Part print with two shaded views. Sizes in mm from the minimum x, y, z corner. Round coordinates to 2 decimals unless told otherwise and drop trailing zeros. Loops run counter-clockwise (first coordinate to the right, second up) from the corner with the lowest first, then second, coordinate; pieces in that order, holes last. Notation, with made-up numbers: M 71,65.25 L 91,65.25 A15 ccw 91,84.25 Z; hole C 63.5,-37.75 d7. An arc over 180 degrees is marked long. Answer as CSV lines item,"result". Start each with the question number.
Item 1: Band-saw the part on B-B (y = 2.2). Count the separate pieces of the cut face and the enclosed holes in it, and give its area (3 significant figures).
Item 2: Wall check: line 1 (X direction, y = 2.4, z = 103.6); line 2 (X direction, y = 2.4, z = 43.5). Give the ranges that are in metal, low to high.
Item 3: Drop flat-ended pins along their axis: pin 1 Ø1 at (x, y) = (100.5, 1.5) entering from +Z; pin 2 Ø1 at (y, z) = (1, 2) entering from -X; pin 3 Ø1 at (y, z) = (2, 99.5) entering from +X; pin 4 Ø3 at (x, z) = (74.45, 51.64) entering from -Y. Give the stop position or say it passes through.
Item 4: Band-saw the part on A-A (x = 47.5). Give the cut face in (y, z).
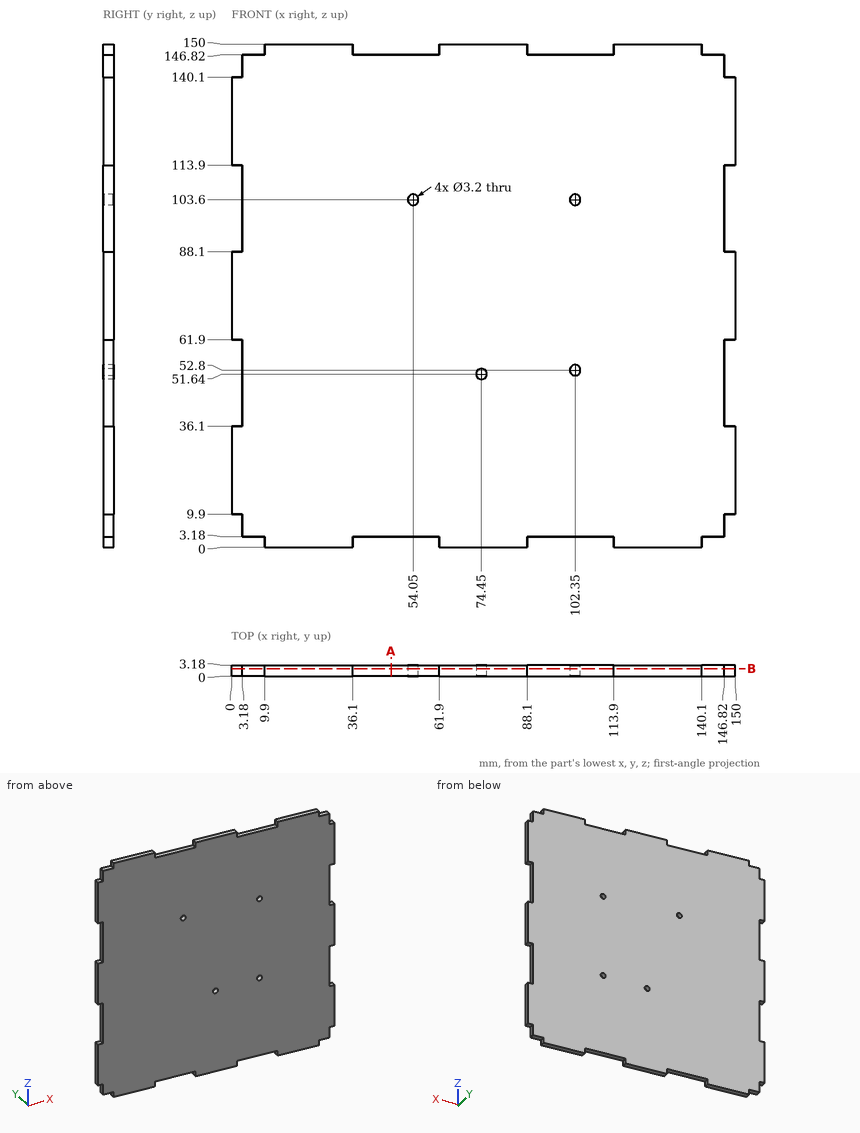
Answer block:
1,separate pieces,"1"
1,enclosed holes,"4"
1,area,"21,600 mm^2"
2,line 1,"x = 3.18 to 52.45, 55.65 to 100.75, 103.95 to 146.82"
2,line 2,"x = 3.18 to 146.82"
3,pin 1,"stops at z = 146.82"
3,pin 2,"stops at x = 9.9"
3,pin 3,"stops at x = 146.82"
3,pin 4,"passes through"
4,outline,"M 0,3.18 L 3.18,3.18 L 3.18,146.82 L 0,146.82 Z"
